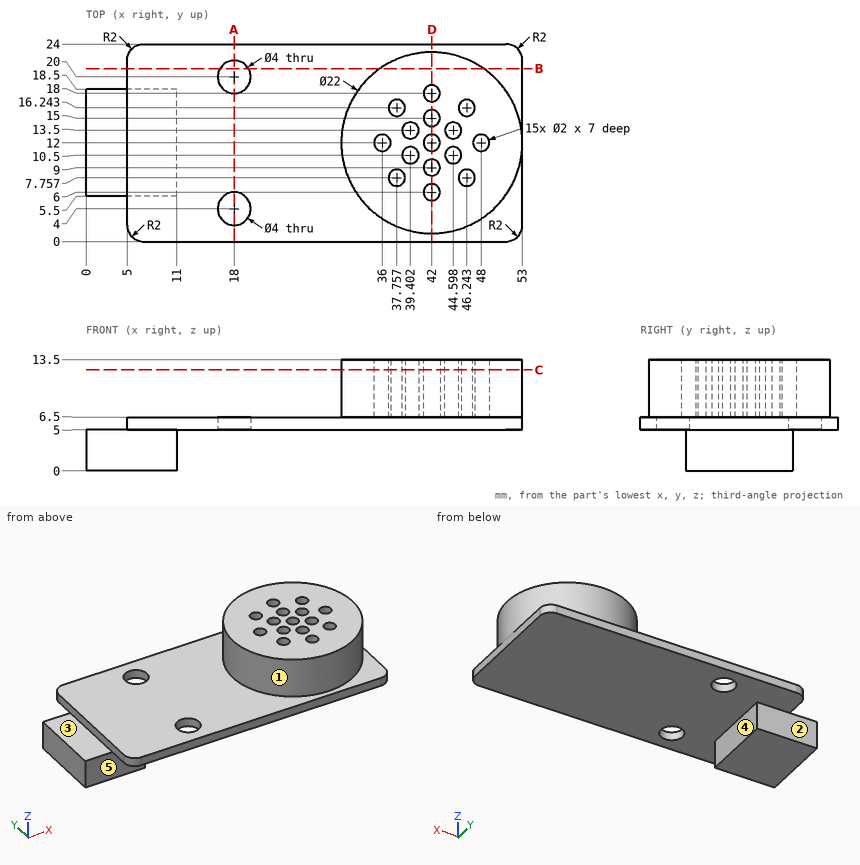
The figure shows three views and two pictorial views of one solid part (mm, origin at its lowest corner). Answer the questions. A direction names the side the tool comes from. Round coordinates to 2 decimals unless told otherwise and drop trailing zeros. Write each loop counter-clockwise with the first axis right and the second up, starting at its lowest first coordinate (ties: lowest second). Pieces come first, ordered by that corner, then holes. Notation, with made-up numbers: (42, 53) - (61, 53) arc R31 ccw to (61, 83) - close; hole circle Ø4 at (-3.5, 89.25). An arc over 180 degrees is marked (long way). Use one line per item in the form item = value. Start each with the question number.
Item 1: A tool of negligible diameter and unlimited length cuts with its end or side. For the marked faces 1, 2, 3, 4 and 5, from which of +Z, -Z, +X, -X, +Y, -Y can it reach the whole face along a straight path? Write none if from no direction.
Item 2: A cutting plane is placed at C-C (z = 12.25). Give the number of separate pieces and of enclosed holes in the cut face, plus the area to 3 significant figures.
Item 3: Find the intervals of material crossed by line 1 (Y direction, x = 42, z = 11); line 2 (X direction, y = 11, z = 2.75); line 3 (Z direction, x = 17, y = 2), in increasing order. Write a range as [from, to].
Item 4: A cutting plane is placed at B-B (y = 21). Write down the section's boundary in (x, z) (1 decimal).
Item 5: Flat-ended cylindrical pins translate along their axes: pin 1 Ø1.2 at (x, y) = (42, 9) entering from -Z; pin 2 Ø2.5 at (x, y) = (2.5, 13.5) entering from +Z; pin 3 Ø2 at (x, y) = (16, 5) entering from +Z. Find the tip coordinate at first contact, or state that the pin passes through.
Item 6: A cutting plane is placed at D-D (x = 42). Write down the section's boundary in (y, z), plus the area to 3 significant figures.
Item 7: A cutting plane is placed at A-A (x = 18). Write down the section's boundary in (y, z).
The answers:
q1.face_1 = +Z
q1.face_2 = -Z, +X, -X, +Y
q1.face_3 = +Z, -X, +Y, -Y
q1.face_4 = -Z, +X, +Y, -Y
q1.face_5 = -Z, +X, -X, -Y
q2.separate_pieces = 1
q2.enclosed_holes = 15
q2.area = 333 mm^2
q3.line_1 = [1, 5], [7, 8], [10, 11], [13, 14], [16, 17], [19, 23]
q3.line_2 = [0, 11]
q3.line_3 = [5, 6.5]
q4.outline = (5, 5) - (16.3, 5) - (16.3, 6.5) - (5, 6.5) - close; (19.7, 5) - (53, 5) - (53, 6.5) - (48.3, 6.5) - (48.3, 13.5) - (35.7, 13.5) - (35.7, 6.5) - (19.7, 6.5) - close
q5.pin_1 = 5
q5.pin_2 = 5
q5.pin_3 = 6.5
q6.outline = (0, 5) - (24, 5) - (24, 6.5) - (23, 6.5) - (23, 13.5) - (19, 13.5) - (19, 6.5) - (17, 6.5) - (17, 13.5) - (16, 13.5) - (16, 6.5) - (14, 6.5) - (14, 13.5) - (13, 13.5) - (13, 6.5) - (11, 6.5) - (11, 13.5) - (10, 13.5) - (10, 6.5) - (8, 6.5) - (8, 13.5) - (7, 13.5) - (7, 6.5) - (5, 6.5) - (5, 13.5) - (1, 13.5) - (1, 6.5) - (0, 6.5) - close
q6.area = 120 mm^2
q7.outline = (0, 5) - (2, 5) - (2, 6.5) - (0, 6.5) - close; (6, 5) - (18, 5) - (18, 6.5) - (6, 6.5) - close; (22, 5) - (24, 5) - (24, 6.5) - (22, 6.5) - close
